Part model, mm, in its own coordinate system. A direction names the side the tool comes from. Round coordinates to 2 decimals unless told otherwise and drop trailing zeros. Loops run counter-clockwise (first coordinate to the right, second up) from the corner with the lowest first, then second, coordinate; pieces in that order, holes last. Notation, with made-up numbers: (-16.75, 67.5) -> (38.25, 67.5) arc R15 ccw to (38.25, 93.5) -> close; hole circle Ø9 at (4.25, 21). An arc over 180 degrees is marked (long way). Use a Markdown table: item, result. Add a question column.
Item 1: Flat gauge pins, fed straight in: pin 1 (10 mm diameter, centred on y = 293.5, z = 25.5, fed in from -X); pin 2 (12 mm diameter, centred on x = -419, y = 173, fed in from +Z); pin 3 (1.5 mm diameter, centred on x = -452, y = 161, fed in from -Z); pin 4 (24 mm diameter, centred on y = -130, z = -130, fed in from -X) (3 decimals). Where does each tip first touch, or does it go through?
Item 2: Probe line 1 (Y direction, x = -6, z = -130); line 2 (Z direction, x = -34, y = -130). List the from-to ranges inside material, lowest first. Write a range as [from, to].
Item 3: Two-plate mould, pull along Z, no slides. Class faces 1 (the face through (-412, 385, -180)), 2 (the face through (-590, 385, 2)), 3 (the face through (-29.72, -144.985, 130.66)), 4 (the face through (-100.7, -43.554, -138.304)): pulls with the +Z half, pulls with the -Z half, needs draft (parallel to the pull), parting line crosses it, or undercut.
Item 4: Cut at D-D, the plane y = 330. List the corners of the cut face in (x, z).
Item 5: Which spindle directions (+Z, -Z, +X, -X, +Y, -Y) get a long thin tool onto all of the face, cutting with end or side? Do faces 5 (the face through (-533, 360, -83)), 6 (the face through (-307.497, 330.98, 22.762)), 7 (the face through (-10, 144, 124)). Say none if no direction does.
Item 6: Cut at A-A, the plane x = -280. State how many separate pieces and enclosed holes the cut face has, plus the area to 3 significant figures.
Item 7: Cut at B-B, the plane x = -128. List the corners of the cut face in (y, z).
```python
from build123d import *

# Parameters (mm, degrees)
SKETCH2_R                 = 145
SKETCH2_R_2               = 105
BOSS_EXTRUDE1_START       = -50
SKETCH3_W                 = 360
SKETCH3_H                 = 360
SKETCH3_R                 = 145
BOSS_EXTRUDE1_DEPTH       = 50
FILLET1_R                 = 10
SKETCH4_W                 = 360
SKETCH4_H                 = 360
SKETCH4_R                 = 145
BOSS_EXTRUDE2_DEPTH       = 50
FILLET2_R                 = 10
SKETCH5_R                 = 30
CUT_EXTRUDE1_DEPTH        = 10
CUT_EXTRUDE2_REACH        = 734.735
SKETCH7_R                 = 15
CIRPATTERN1_COUNT         = 4
SKETCH8_R                 = 30
CUT_EXTRUDE3_DEPTH        = 10
SKETCH9_R                 = 15
CUT_EXTRUDE4_DEPTH        = 847.69947443
CIRPATTERN4_START         = 360
CIRPATTERN4_OUTLINE_R     = 15
CIRPATTERN4_DEPTH         = 50
CIRPATTERN4_START_2       = 400
CIRPATTERN4_2_OUTLINE_R   = 30
CIRPATTERN4_2_OUTLINE_R_2 = 15
CIRPATTERN4_2_DEPTH       = 10
CHAMFER1_SIZE             = 10
CHAMFER2_SIZE             = 10


# Read off the part's stored shape, not the designer's step: CirPattern4
with BuildPart() as part:
    # Sweep-Thin1: sweep along a path in Sketch1
    with BuildLine(Plane.XY) as sweep_thin1_path:
        Line((0, 0), (-150, 0))
        ThreePointArc((-150, 0), (-333.847763109, 76.152236891), (-410, 260))
        Line((-410, 260), (-410, 410))
    # Sketch2 → Sweep-Thin1 (sweep)
    with BuildSketch(Plane(origin=(0, 0, 0), x_dir=(0, 0, -1), z_dir=(1, 0, 0))):
        Circle(SKETCH2_R)
        Circle(SKETCH2_R_2, mode=Mode.SUBTRACT)
    sweep(path=sweep_thin1_path.line)

    # Sketch3 → Boss-Extrude1 (add)
    with BuildSketch(Plane(origin=(0, 0, 0), x_dir=(0, 0, -1), z_dir=(1, 0, 0)).offset(BOSS_EXTRUDE1_START)):
        Rectangle(SKETCH3_W, SKETCH3_H)
        with Locations(Location((0, 0, 0), (0, 0, 270))):
            Circle(SKETCH3_R, mode=Mode.SUBTRACT)
    extrude(amount=BOSS_EXTRUDE1_DEPTH)

    # Fillet1
    fillet1_edges = [part.edges().sort_by_distance(p)[0] for p in [
        (-25, 180, -180),
        (-25, -180, -180),
        (-25, -180, 180),
        (-25, 180, 180),
    ]]
    fillet(fillet1_edges, radius=FILLET1_R)

    # Sketch4 → Boss-Extrude2 (add)
    with BuildSketch(Plane(origin=(0, 410, 0), x_dir=(1, 0, 0), z_dir=(0, 1, 0))):
        with Locations((-410, 0)):
            Rectangle(SKETCH4_W, SKETCH4_H)
        with Locations(Location((-410, 0, 0), (0, 0, 180))):
            Circle(SKETCH4_R, mode=Mode.SUBTRACT)
    extrude(amount=-BOSS_EXTRUDE2_DEPTH)

    # Fillet2
    fillet2_edges = [part.edges().sort_by_distance(p)[0] for p in [
        (-230, 385, -180),
        (-230, 385, 180),
        (-590, 385, 180),
        (-590, 385, -180),
    ]]
    fillet(fillet2_edges, radius=FILLET2_R)

    # Sketch5 → Cut-Extrude1 (cut)
    with BuildSketch(Plane(origin=(0, 0, 0), x_dir=(0, 0, -1), z_dir=(1, 0, 0))):
        with Locations((-130, 130)):
            Circle(SKETCH5_R)
    cut_extrude1 = extrude(amount=-CUT_EXTRUDE1_DEPTH, mode=Mode.SUBTRACT)

    # Sketch7 → Cut-Extrude2 (cut, up to next)
    with BuildSketch(Plane(origin=(-10, 0, 0), x_dir=(0, 0, -1), z_dir=(1, 0, 0)), mode=Mode.PRIVATE) as cut_extrude2_sk1:
        with Locations((-130, 130)):
            Circle(SKETCH7_R)
    cut_extrude2_tool1 = extrude(cut_extrude2_sk1.sketch, amount=-CUT_EXTRUDE2_REACH, mode=Mode.PRIVATE) & part.part
    cut_extrude2 = cut_extrude2_tool1.solids().sort_by_distance((-10, 130, 130))[0]
    add(cut_extrude2, mode=Mode.SUBTRACT)

    # CirPattern1: Cut-Extrude1, Cut-Extrude2 ×4 about axis
    cirpattern1_axis = Axis((0, 0, 0), (1, 0, 0))
    add([cut_extrude1.rotate(cirpattern1_axis, i * 360 / CIRPATTERN1_COUNT) for i in range(1, CIRPATTERN1_COUNT)], mode=Mode.SUBTRACT)
    add([cut_extrude2.rotate(cirpattern1_axis, i * 360 / CIRPATTERN1_COUNT) for i in range(1, CIRPATTERN1_COUNT)], mode=Mode.SUBTRACT)

    # Sketch8 → Cut-Extrude3 (cut)
    with BuildSketch(Plane(origin=(0, 410, 0), x_dir=(1, 0, 0), z_dir=(0, 1, 0))):
        with Locations(Location((-540, 130, 0), (0, 0, 180))):
            Circle(SKETCH8_R)
    extrude(amount=-CUT_EXTRUDE3_DEPTH, mode=Mode.SUBTRACT)

    # Sketch9 → Cut-Extrude4 (cut, through all)
    with BuildSketch(Plane(origin=(0, 400, 0), x_dir=(1, 0, 0), z_dir=(0, 1, 0))):
        with Locations(Location((-540, 130, 0), (0, 0, 180))):
            Circle(SKETCH9_R)
    extrude(amount=-CUT_EXTRUDE4_DEPTH, mode=Mode.SUBTRACT)

    # CirPattern4 outline → CirPattern4 (cut)
    with BuildSketch(Plane(origin=(0, 0, 0), x_dir=(1, 0, 0), z_dir=(0, 1, 0)).offset(CIRPATTERN4_START)):
        with Locations((-280, 130)):
            Circle(CIRPATTERN4_OUTLINE_R)
        with Locations((-280, -130)):
            Circle(CIRPATTERN4_OUTLINE_R)
        with Locations((-540, -130)):
            Circle(CIRPATTERN4_OUTLINE_R)
    extrude(amount=CIRPATTERN4_DEPTH, mode=Mode.SUBTRACT)

    # CirPattern4 2 outline → CirPattern4 2 (cut)
    # profile 1 of 3: a face of its own
    with BuildSketch(Plane(origin=(0, 0, 0), x_dir=(1, 0, 0), z_dir=(0, 1, 0)).offset(CIRPATTERN4_START_2)):
        with Locations((-280, 130)):
            Circle(CIRPATTERN4_2_OUTLINE_R)
        with Locations((-280, 130)):
            Circle(CIRPATTERN4_2_OUTLINE_R_2, mode=Mode.SUBTRACT)
    # profile 2 of 3: a face of its own
    with BuildSketch(Plane(origin=(0, 0, 0), x_dir=(1, 0, 0), z_dir=(0, 1, 0)).offset(CIRPATTERN4_START_2)):
        with Locations((-280, -130)):
            Circle(CIRPATTERN4_2_OUTLINE_R)
        with Locations((-280, -130)):
            Circle(CIRPATTERN4_2_OUTLINE_R_2, mode=Mode.SUBTRACT)
    # profile 3 of 3: a face of its own
    with BuildSketch(Plane(origin=(0, 0, 0), x_dir=(1, 0, 0), z_dir=(0, 1, 0)).offset(CIRPATTERN4_START_2)):
        with Locations((-540, -130)):
            Circle(CIRPATTERN4_2_OUTLINE_R)
        with Locations((-540, -130)):
            Circle(CIRPATTERN4_2_OUTLINE_R_2, mode=Mode.SUBTRACT)
    extrude(amount=CIRPATTERN4_2_DEPTH, mode=Mode.SUBTRACT)

    # Chamfer1
    chamfer1_edges = [part.edges().sort_by_distance(p)[0] for p in [
        (0, 0, 105),
    ]]
    chamfer(chamfer1_edges, length=CHAMFER1_SIZE)

    # Chamfer2
    chamfer2_edges = [part.edges().sort_by_distance(p)[0] for p in [
        (-410, 410, 105),
    ]]
    chamfer(chamfer2_edges, length=CHAMFER2_SIZE)


solid = part.part
```
A:
| question | item | result |
|---|---|---|
| 1 | pin 1 | stops at x = -553.54 |
| 1 | pin 2 | stops at z = 144.03 |
| 1 | pin 3 | stops at z = -133.3 |
| 1 | pin 4 | passes through |
| 2 | line 1 | y = [-180, -160], [-100, 100], [160, 180] |
| 2 | line 2 | z = [-180, -145], [-115, 115], [145, 180] |
| 3 | face 1 | pulls with the -Z half |
| 3 | face 2 | needs draft |
| 3 | face 3 | undercut |
| 3 | face 4 | parting line crosses it |
| 4 | outline | circle Ø290 at (-410, 0); hole circle Ø210 at (-410, 0) |
| 5 | face 5 | none |
| 5 | face 6 | +Y |
| 5 | face 7 | +X |
| 6 | separate pieces | 3 |
| 6 | enclosed holes | 1 |
| 6 | area | 71,600 mm^2 |
| 7 | outline | circle Ø290 at (0, 0); hole circle Ø210 at (0, 0) |
